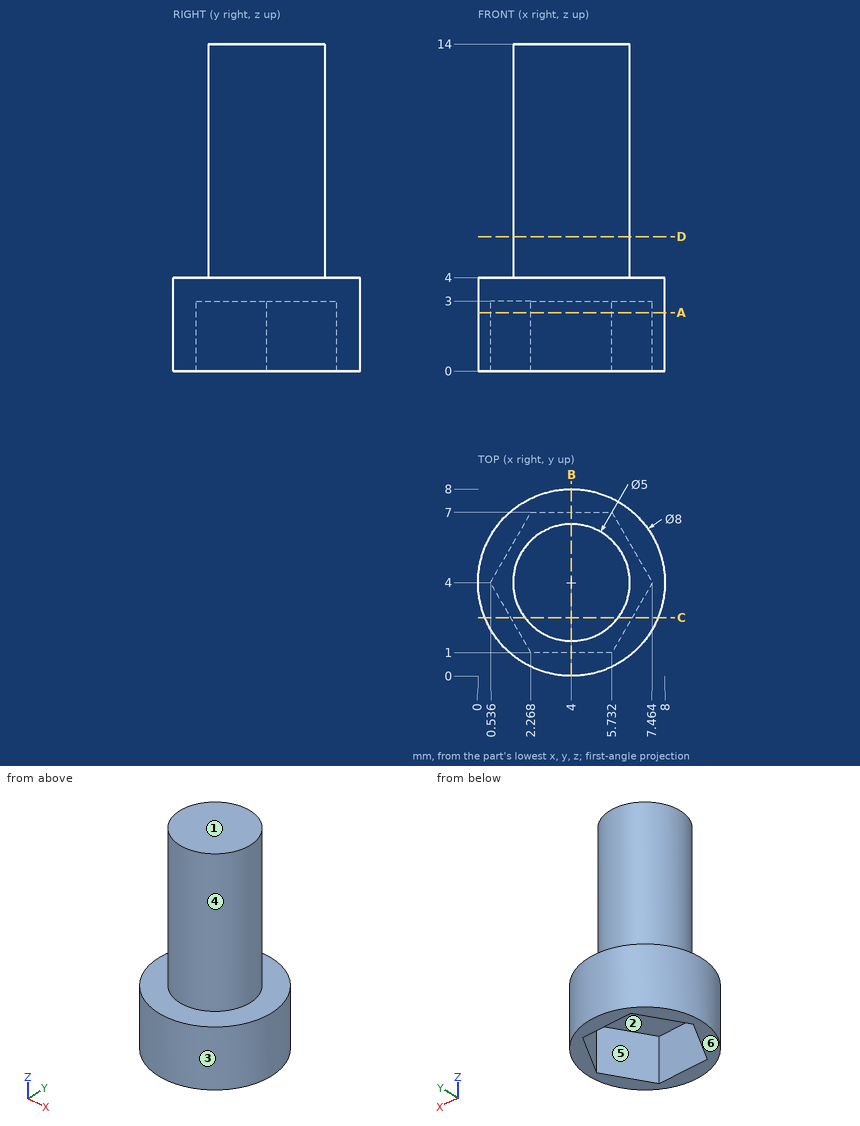
Study the drawing (mm; zero at the part's minimum x, y, z) and answer. A direction names the side the tool comes from. Coordinates: 2 decimals unless noted, no trailing zeros. Write each loop counter-clockwise with the first axis right and the second up, starting at its lowest first coordinate (ties: lowest second). Pieces come first, ordered by that corner, then holes. Notation, with made-up numbers: (24.25, 52.5) - (38.25, 52.5) arc R29 cw to (38.25, 77.5) - close; hole circle Ø2 at (2.25, -28.5). An arc over 180 degrees is marked (long way). Answer as a JSON object with one key per item and string values. Group by question number.
1. A cutting plane is placed at B-B (x = 4). Determine the outline of the cut face in (y, z), plus the area to 3 significant figures.
2. Consider L1, parallel to Z at x = 1.25, y = 6.25; L2, parallel to Z at x = 4.5, y = 6.5; L3, parallel to Y at x = 6.5, z = 1. Determine where each line is inside the solid, lowest interval first. Write a range as [from, to].
3. The mould has two halves that part along Y. Classify the marked faces 1, 2 and 3: +Y half, -Y half, draft (parallel to the pull), parting line (faces both ways), or undercut.
4. Each of these flat-tipped pins is pushed along its axis until it touches: P1, Ø1.5, axis at x = 7, z = 6, coming from the -Y side; P2, Ø3, axis at x = 6, z = 11.5, coming from the +Y side; P3, Ø1.8, axis at x = 5.5, y = 4.5, coming from the -Z side. Where does it stop, or does it pass through?
5. A cutting plane is placed at D-D (z = 5.75). Determine the outline of the cut face in (x, y), plus the area to 3 significant figures.
6. A cutting plane is placed at A-A (z = 2.5). Determine the outline of the cut face in (x, y), plus the area to 3 significant figures.
7. Which of the six approach directions +Z, -Z, +X, -X, +Y, -Y give full straight-line access (tool end or side, diameter ignored) to the marked faces 4, 5 and 6?
8. A cutting plane is placed at C-C (y = 2.5). Determine the outline of the cut face in (x, z).
Worked out:
{
 "1": {"outline": "(0, 0) - (1, 0) - (1, 3) - (7, 3) - (7, 0) - (8, 0) - (8, 4) - (6.5, 4) - (6.5, 14) - (1.5, 14) - (1.5, 4) - (0, 4) - close", "area": "64.0 mm²"},
 "2": {"L1": "z = [0, 4]", "L2": "z = [3, 4]", "L3": "y = [0.88, 2.33], [5.67, 7.12]"},
 "3": {"face 1": "draft", "face 2": "undercut", "face 3": "parting line"},
 "4": {"P1": "stops at y = 2.91", "P2": "stops at y = 6.45", "P3": "stops at z = 3"},
 "5": {"outline": "circle Ø5 at (4, 4)", "area": "19.6 mm²"},
 "6": {"outline": "circle Ø8 at (4, 4); hole (0.54, 4) - (2.27, 1) - (5.73, 1) - (7.46, 4) - (5.73, 7) - (2.27, 7) - close", "area": "19.1 mm²"},
 "7": {"face 4": "+Z", "face 5": "-Z", "face 6": "-Z, +X, -X, +Y, -Y"},
 "8": {"outline": "(0.29, 0) - (1.4, 0) - (1.4, 3) - (6.6, 3) - (6.6, 0) - (7.71, 0) - (7.71, 4) - (6, 4) - (6, 14) - (2, 14) - (2, 4) - (0.29, 4) - close"}
}
